Autodesk Inventor part; units mm, degrees
ref_plane "YZ Plane" through (0, 0, 0) normal (1, 0, 0) x (0, 1, 0)
ref_plane "XZ Plane" through (0, 0, 0) normal (0, 1, 0) x (-1, 0, 0)
ref_plane "XY Plane" through (0, 0, 0) normal (0, 0, 1) x (1, 0, 0)
sketch "Sketch1" plane through (0, 0, 0) normal (0, 1, 0) x (-1, 0, 0)
  arc A0 (11.4671, -0.8698) -> (-11.4671, -0.8698) centre (0, 0) ccw
  arc A1 (-5.9828, -73.1731) -> (5.9828, -73.1731) centre (0, -72.7193) ccw
  line L0 (11.4671, -0.8698) -> (5.9828, -73.1731)
  line L1 (-5.9828, -73.1731) -> (-11.4671, -0.8698)
  line L2 (7.2791, -73.2714) -> (12.7633, -0.9681)
  arc A2 (12.7633, -0.9681) -> (-12.7633, -0.9681) centre (0, 0) ccw
  line L3 (-12.7633, -0.9681) -> (-7.2791, -73.2714)
  arc A3 (-7.2791, -73.2714) -> (7.2791, -73.2714) centre (0, -72.7193) ccw
  dimension "d0" = 23
  dimension "d1" = 12
  dimension "d2" = 72.511
  dimension "d6" = 1.3
extrude "Extrusion1" add sketch "Sketch1" along normal blind 6
properties part number "tandriem32Tnaar16T_lengte200"
Check sheet for the modelled part. Datum: model origin and axes. Units: mm. A direction names the side the tool comes from. Coordinates: 2 decimals unless noted, no trailing zeros. Loops run counter-clockwise (first coordinate to the right, second up) from the corner with the lowest first, then second, coordinate; pieces in that order, holes last. Notation, with made-up numbers: (30.25, 54) -> (52.25, 54) arc R35 ccw to (52.25, 88) -> close; hole circle Ø11 at (7.5, -31.5). An arc over 180 degrees is marked (long way). Answer in a Markdown table with one row per item.
1. Sectioned sample at B-B, the plane y = 4.15. Record the boundary of the cut face in (x, z).
Check values:
| item | result |
|---|---|
| outline | (-12.76, -0.97) -> (-7.28, -73.27) arc R7.3 ccw to (7.28, -73.27) -> (12.76, -0.97) arc R12.8 ccw (long way) to start; hole (-11.47, -0.87) -> (-5.98, -73.17) arc R6 ccw to (5.98, -73.17) -> (11.47, -0.87) arc R11.5 ccw (long way) to start |
2. Sectioned sample at C-C, the plane x = 2. Record the boundary of the cut face in (y, z), then the cut area to 3 significant figures.
Check values:
| item | result |
|---|---|
| outline | (0, -79.74) -> (6, -79.74) -> (6, -78.38) -> (0, -78.38) -> close; (0, 11.32) -> (6, 11.32) -> (6, 12.64) -> (0, 12.64) -> close |
| area | 16.1 mm2 |
3. Go/stop test with flat-tipped pins: pin 1 (1 mm diameter, centred on x = 7, y = 4, fed in from +Z); pin 2 (2 mm diameter, centred on y = 5, z = -45.5, fed in from +X). Record where each tip stops, or that it passes through.
Check values:
| item | result |
|---|---|
| pin 1 | stops at z = 11.03 |
| pin 2 | stops at x = 9.46 |
4. Access from +Z, -Z, +X, -X, +Y, -Y to the whole of each face (thin tool, end or side, straight path). Record for faces 1 (the face through (0.265, 2.958, 11.497)), 2 (the face through (10, 6, -33)).
Check values:
| item | result |
|---|---|
| face 1 | +Y, -Y |
| face 2 | +Z, -Z, +X, -X, +Y |
5. Release check for a two-part mould opening along Z. For faces 3 (the face through (-0.153, 2.958, -80.018)), 4 (the face through (10, 0, -33)), 5 (the face through (8.687, 2.958, -37.528)) record: released by +Z, released by -Z, zero draft, split by the parting line, or undercut.
Check values:
| item | result |
|---|---|
| face 3 | released by -Z |
| face 4 | zero draft |
| face 5 | undercut |
6. Sectioned sample at A-A, the plane z = 0. Record the boundary of the cut face in (x, y).
Check values:
| item | result |
|---|---|
| outline | (-12.8, 0) -> (-11.5, 0) -> (-11.5, 6) -> (-12.8, 6) -> close; (11.5, 0) -> (12.8, 0) -> (12.8, 6) -> (11.5, 6) -> close |
7. Material ranges on line 1 along X through (y, z) = (5.1, 0); line 2 along Z through (x, y) = (0.5, 4.45); line 3 along X through (y, z) = (3.15, 7), recorded low to high. Write a range as [from, to].
Check values:
| item | result |
|---|---|
| line 1 | x = [-12.8, -11.5], [11.5, 12.8] |
| line 2 | z = [-80, -78.7], [11.49, 12.79] |
| line 3 | x = [-10.72, -9.12], [9.12, 10.72] |
